For this review, take the finished solid that the model builds, in its own axes (mm). A direction names the side the tool comes from. Coordinates: 2 decimals unless noted, no trailing zeros. Order: outer loops, then holes, each group sorted by start corner. A loop starts at its lowest first (then second) coordinate and runs counter-clockwise, first axis right, second up.
from build123d import *

# Parameters (mm, degrees)
BOSS_EXTRUDE1_DEPTH     = 6.499999954
CIRPATTERN1_COUNT       = 20
SKETCH2_W               = 10.342329408
SKETCH2_H               = 1.5875
CUT_EXTRUDE1_DEPTH      = 17.713324345
CUT_EXTRUDE1_DEPTH_BACK = 17.713324345
SKETCH3_R               = 1.6
SKETCH4_R               = 13.77
BOSS_EXTRUDE2_DEPTH     = 3.30250003
CUT_EXTRUDE2_DEPTH      = 13.208


with BuildPart() as part:
    # Sketch1 → Boss-Extrude1 (new, symmetric)
    with BuildSketch(Plane(origin=(0, 0, 0), x_dir=(1, 0, 0), z_dir=(0, 1, 0))):
        with BuildLine():
            ThreePointArc((0.872060607, 8.659786465), (0.562967303, 8.148255135), (0, 7.947579308))
            ThreePointArc((0, 7.947579308), (-1.243275317, -7.849731418), (2.45593707, 7.55859709))
            ThreePointArc((2.45593707, 7.55859709), (1.982535589, 7.923417607), (1.846642263, 8.505427895))
            ThreePointArc((1.846642263, 8.505427895), (1.749626992, 8.862101959), (1.434119122, 9.054671776))
            ThreePointArc((1.434119122, 9.054671776), (1.074545959, 8.969024291), (0.872060607, 8.659786465))
        make_face()
    boss_extrude1 = extrude(amount=BOSS_EXTRUDE1_DEPTH, both=True)

    # CirPattern1: Boss-Extrude1 ×20 about axis
    cirpattern1_axis = Axis((0, 0, 0), (0, 1, 0))
    for i in range(1, CIRPATTERN1_COUNT):
        add(boss_extrude1.rotate(cirpattern1_axis, i * 360 / CIRPATTERN1_COUNT))

    # Sketch2 → Revolve3 (revolve)
    with BuildSketch(Plane(origin=(0, 0, 0), x_dir=(0, 0, -1), z_dir=(1, 0, 0)), mode=Mode.PRIVATE) as revolve3_sk:
        with Locations((5.171164704, 7.293749954)):
            Rectangle(SKETCH2_W, SKETCH2_H)
    revolve(revolve3_sk.sketch.rotate(Axis((0, 3.3, 0), (0, -1, 0)), 180), axis=Axis((0, 3.3, 0), (0, -1, 0)))

    # Sketch3 → Cut-Extrude1 (cut, two sides: drawn at the far end of the back side and taken through both)
    with BuildSketch(Plane(origin=(0, 0, 0), x_dir=(-1, 0, 0), z_dir=(0, -1, 0)).offset(-CUT_EXTRUDE1_DEPTH_BACK)):
        with Locations(Location((0, 0, 0), (0, 0, 90))):
            Circle(SKETCH3_R)
    extrude(amount=CUT_EXTRUDE1_DEPTH + CUT_EXTRUDE1_DEPTH_BACK, mode=Mode.SUBTRACT)

    # Sketch4 → Boss-Extrude2 (add)
    with BuildSketch(Plane(origin=(0, -9.802499984, 0), x_dir=(1, 0, 0), z_dir=(0, 1, 0))):
        with Locations(Location((0, 0, 0), (0, 0, 270))):
            Circle(SKETCH4_R)
    extrude(amount=BOSS_EXTRUDE2_DEPTH)

    # Sketch5 → Cut-Extrude2 (cut)
    with BuildSketch(Plane(origin=(0, -9.802499984, 0), x_dir=(1, 0, 0), z_dir=(0, 1, 0))):
        Polygon((-2.917259676, 4.661702584), (-5.495782701, -0.195569697), (-2.578523025, -4.857272281), (2.917259676, -4.661702584), (5.495782701, 0.195569697), (2.578523025, 4.857272281), align=None)
    extrude(amount=CUT_EXTRUDE2_DEPTH, mode=Mode.SUBTRACT)


solid = part.part
1. Take a section at D-D, the plane x = -7. Give the boundary of the cut face in (y, z).
Answer below:
outline: (-9.8, -11.86) - (-6.5, -11.86) - (-6.5, -4.32) - (6.5, -4.32) - (6.5, -7.61) - (8.09, -7.61) - (8.09, 7.61) - (6.5, 7.61) - (6.5, 4.32) - (-6.5, 4.32) - (-6.5, 11.86) - (-9.8, 11.86) - close
2. The part is to be moulded in two halves that separate along Z. For faces 1 (the face through (-0.455, 7.305, -10.332)), 2 (the face through (4.188, -3.291, 2.267)), 3 (the face through (0, -9.802, 6)), say which applies: +Z half, -Z half, draft (parallel to the pull), parting line (faces both ways), or undercut.
Answer below:
face 1: parting line
face 2: undercut
face 3: draft
3. Machinability: for faces 4 (the face through (-4.188, -3.291, -2.267)), 5 (the face through (2, 8.087, 0)), 6 (the face through (-9, -6.5, 0)), which of the approach directions +Z, -Z, +X, -X, +Y, -Y give a long, thin tool a straight path to every point of the face, cutting with its end or side? Answer none if there is none.
Answer below:
face 4: -Y
face 5: +Z, -Z, +X, -X, +Y
face 6: none
4. Take a section at C-C, the plane x = 9.5. Give the boundary of the cut face in (y, z), plus the area to 3 significant figures.
Answer below:
outline: (-9.8, -9.97) - (-6.5, -9.97) - (-6.5, 9.97) - (-9.8, 9.97) - close; (6.5, -4.09) - (8.09, -4.09) - (8.09, 4.09) - (6.5, 4.09) - close
area: 78.8 mm2
5. Take a section at A-A, the plane y = -8.5. Give the boundary of the cut face in (x, z), plus the area to 3 significant figures.
Answer below:
outline: circle Ø27.54 at (0, 0); hole (-5.5, 0.2) - (-2.92, -4.66) - (2.58, -4.86) - (5.5, -0.2) - (2.92, 4.66) - (-2.58, 4.86) - close
area: 517 mm2
6. To check wall thickness, follow L1, parallel to X at y = 6.55, z = 0; L2, parallel to Y at x = 9.5, z = -4; L3, parallel to Y at x = -11.25, z = 7.5. State the ranges of each line that lie inside material, in increasing order.
Answer below:
L1: x = -10.34 to -1.6, 1.6 to 10.34
L2: y = -9.8 to -6.5, 6.5 to 8.09
L3: y = -9.8 to -6.5
7. Take a section at B-B, the plane z = -5.25. Give the boundary of the cut face in (x, y), plus the area to 3 significant figures.
Answer below:
outline: (-12.73, -9.8) - (12.73, -9.8) - (12.73, -6.5) - (6.26, -6.5) - (6.26, 6.5) - (8.91, 6.5) - (8.91, 8.09) - (-8.91, 8.09) - (-8.91, 6.5) - (-6.26, 6.5) - (-6.26, -6.5) - (-12.73, -6.5) - close
area: 275 mm2
8. Clearance check with flat-ended pins moving along their axes: pin 1 Ø3 at (y, z) = (-5.5, 10) entering from -X; pin 2 Ø2 at (y, z) = (-4.5, 4.5) entering from +X; pin 3 Ø16.5 at (x, z) = (4, 0) entering from -Y; pin 4 Ø3 at (x, y) = (-0.5, 5.5) entering from -Z. State where each tip first meets the part, or that it passes through.
Answer below:
pin 1: stops at x = -10.52
pin 2: stops at x = 8.22
pin 3: stops at y = -9.8
pin 4: stops at z = -10.34
